```python
from build123d import *
from build123d.topology import SkipClean

# Parameters (mm, degrees)
BOSS_EXTRUDE1_DEPTH     = 2.5
BOSS_EXTRUDE1_2_DEPTH   = 2.5
BOSS_EXTRUDE2_DEPTH     = 6.35
BOSS_EXTRUDE3_DEPTH     = 6.35
SKETCH4_R               = 3.175
CUT_EXTRUDE1_DEPTH      = 25.4
SKETCH5_R               = 1.5875
CUT_EXTRUDE2_DEPTH      = 25.4
CUT_EXTRUDE3_DEPTH      = 25.4
CUT_EXTRUDE4_REACH      = 43
CUT_EXTRUDE4_END_RADIUS = 3.175
CUT_EXTRUDE5_REACH      = 39.36
SKETCH8_W               = 2.54
SKETCH8_H               = 9.525
SKETCH9_W               = 0.7112
SKETCH9_H               = 15.2
BOSS_EXTRUDE4_DEPTH     = 17
BOSS_EXTRUDE5_DEPTH     = 1.016
SKETCH11_W              = 1.176658287
SKETCH11_H              = 2.5
SKETCH11_W_2            = 2.636987944
SKETCH11_H_2            = 15.2
BOSS_EXTRUDE6_DEPTH     = 1.27
CUT_EXTRUDE6_DEPTH      = 38.864332241
BOSS_EXTRUDE7_START     = 2.54
BOSS_EXTRUDE7_DEPTH     = 2.54
BOSS_EXTRUDE8_DEPTH     = 2.54
BOSS_EXTRUDE9_DEPTH     = 0.508
BOSS_EXTRUDE10_DEPTH    = 0.508
CUT_EXTRUDE7_DEPTH      = 3.81
CUT_EXTRUDE8_DEPTH      = 3.81
BOSS_EXTRUDE11_DEPTH    = 3.81
BOSS_EXTRUDE12_START    = -10.16
SKETCH21_W              = 49.554714962
SKETCH21_H              = 15.2
SKETCH21_R              = 3.175
BOSS_EXTRUDE12_DEPTH    = 10.16


with BuildPart() as part:
    # Sketch1 → Boss-Extrude1 (new body)
    with BuildSketch(Plane.XY):
        Polygon((5.08, 0), (0, 0), (0, 19.141079028), (-1.033059908, 19.141079028), (-3.75575709, 23.125698967), (-8.376397661, 9.077684872), (-11.679025045, 6.820994294), (-21.26996, 20.857160675), (-22.86, 19.770683798), (-22.86, -3.81), (8.89, -3.81), (8.89, 24.384), (5.08, 24.384), align=None)
    extrude(amount=BOSS_EXTRUDE1_DEPTH)



with BuildPart() as body_2:
    # Sketch1 → Boss-Extrude1 2 (new body)
    with BuildSketch(Plane.XY):
        Polygon((-10.069369191, 23.749), (-4.328956497, 23.964566322), (-4.615556201, 24.384), (-16.108492032, 24.384), (-17.03780348, 23.749), align=None)
    extrude(amount=BOSS_EXTRUDE1_2_DEPTH)


with BuildPart() as part_1:
    add(part.part)

    add(body_2.part)  # Boss-Extrude2 merges body 2
    # Sketch2 → Boss-Extrude2 (add)
    with BuildSketch(Plane.XY.offset(2.5)):
        Polygon((-11.679025045, 6.820994294), (-21.26996, 20.857160675), (-22.86, 19.770683798), (-22.86, -3.81), (8.89, -3.81), (8.89, 24.384), (5.08, 24.384), (5.08, 0), (0, 0), (0, 19.141079028), (-1.033059908, 19.141079028), (-3.75575709, 23.125698967), (-8.376397661, 9.077684872), align=None)
        Polygon((-16.108492032, 24.384), (-18.00931945, 23.085161582), (-8.418384495, 9.048995201), (-8.376397661, 9.077684872), (-3.75575709, 23.125698967), (-1.033059908, 19.141079028), (0, 19.141079028), (0, 0), (5.08, 0), (5.08, 24.384), align=None)
    extrude(amount=BOSS_EXTRUDE2_DEPTH)

    # Sketch3 → Boss-Extrude3 (add)
    with BuildSketch(Plane(origin=(0, 0, 0), x_dir=(-1, 0, 0), z_dir=(0, 0, -1))):
        Polygon((-8.89, 24.384), (-8.89, -3.81), (22.86, -3.81), (22.86, 19.770683798), (21.26996, 20.857160675), (11.679025045, 6.820994294), (8.376397661, 9.077684872), (18.00931945, 23.085161582), (16.108492032, 24.384), align=None)
    extrude(amount=BOSS_EXTRUDE3_DEPTH)

    # Sketch4 → Cut-Extrude1 (cut)
    with BuildSketch(Plane(origin=(0, 24.384, 0), x_dir=(1, 0, 0), z_dir=(0, 1, 0))):
        with Locations(Location((2.54, -1.25, 0), (0, 0, 270))):
            Circle(SKETCH4_R)
    extrude(amount=-CUT_EXTRUDE1_DEPTH, mode=Mode.SUBTRACT)

    # Sketch5 → Cut-Extrude2 (cut)
    with BuildSketch(Plane(origin=(0, -1.016, 0), x_dir=(1, 0, 0), z_dir=(0, 1, 0))):
        with Locations(Location((2.54, -1.25, 0), (0, 0, 270))):
            Circle(SKETCH5_R)
    extrude(amount=-CUT_EXTRUDE2_DEPTH, mode=Mode.SUBTRACT)

    # Sketch6 → Cut-Extrude3 (cut)
    with BuildSketch(Plane.XY.offset(8.85)):
        Polygon((-22.86, 16.430904611), (-9.029357481, -3.81), (-22.86, -3.81), align=None)
    extrude(amount=-CUT_EXTRUDE3_DEPTH, mode=Mode.SUBTRACT)

    # Cut-Extrude4: up to this cylinder (the profile starts outside it)
    with SkipClean():  # the faces are left unmerged after this step: merging them gives an invalid solid
        cut_extrude4_end = Plane(origin=(2.54, 2.159, 1.25), z_dir=(0, 1, 0)) * Cylinder(CUT_EXTRUDE4_END_RADIUS, 96.045024, mode=Mode.PRIVATE)
        # Sketch7 → Cut-Extrude4 (cut, up to the surface)
        with BuildSketch(Plane(origin=(8.89, 0, 0), x_dir=(0, 0, -1), z_dir=(1, 0, 0)), mode=Mode.PRIVATE) as cut_extrude4_sk1:
            with BuildLine():
                ThreePointArc((1.925, 2.159), (-1.25, 5.334), (-4.425, 2.159))
                Line((-4.425, 2.159), (1.925, 2.159))
            make_face()
        cut_extrude4_tool1 = extrude(cut_extrude4_sk1.sketch, amount=-CUT_EXTRUDE4_REACH, mode=Mode.PRIVATE) - cut_extrude4_end
        add(cut_extrude4_tool1.solids().sort_by_distance((8.89, 3.506512, 1.25))[0], mode=Mode.SUBTRACT)
        # Sketch7 → Cut-Extrude4 (cut, up to the surface)
        with BuildSketch(Plane(origin=(8.89, 0, 0), x_dir=(0, 0, -1), z_dir=(1, 0, 0)), mode=Mode.PRIVATE) as cut_extrude4_sk2:
            with BuildLine():
                Line((1.925, 2.159), (-4.425, 2.159))
                ThreePointArc((-4.425, 2.159), (-3.49506403, -0.08606403), (-1.25, -1.016))
                ThreePointArc((-1.25, -1.016), (0.99506403, -0.08606403), (1.925, 2.159))
            make_face()
        cut_extrude4_tool2 = extrude(cut_extrude4_sk2.sketch, amount=-CUT_EXTRUDE4_REACH, mode=Mode.PRIVATE) - cut_extrude4_end
        add(cut_extrude4_tool2.solids().sort_by_distance((8.89, 0.811488, 1.25))[0], mode=Mode.SUBTRACT)
        # Sketch7 → Cut-Extrude4 (cut, up to the surface)
        with BuildSketch(Plane(origin=(8.89, 0, 0), x_dir=(0, 0, -1), z_dir=(1, 0, 0)), mode=Mode.PRIVATE) as cut_extrude4_sk3:
            with BuildLine():
                ThreePointArc((1.925, 2.159), (-1.25, 5.334), (-4.425, 2.159))
                Line((-4.425, 2.159), (1.925, 2.159))
            make_face()
        cut_extrude4_tool3 = extrude(cut_extrude4_sk3.sketch, amount=-CUT_EXTRUDE4_REACH, mode=Mode.PRIVATE) - cut_extrude4_end
        add(cut_extrude4_tool3.solids().sort_by_distance((8.89, 3.506512, 1.25))[0], mode=Mode.SUBTRACT)
        # Sketch7 → Cut-Extrude4 (cut, up to the surface)
        with BuildSketch(Plane(origin=(8.89, 0, 0), x_dir=(0, 0, -1), z_dir=(1, 0, 0)), mode=Mode.PRIVATE) as cut_extrude4_sk4:
            with BuildLine():
                Line((1.925, 2.159), (-4.425, 2.159))
                ThreePointArc((-4.425, 2.159), (-3.49506403, -0.08606403), (-1.25, -1.016))
                ThreePointArc((-1.25, -1.016), (0.99506403, -0.08606403), (1.925, 2.159))
            make_face()
        cut_extrude4_tool4 = extrude(cut_extrude4_sk4.sketch, amount=-CUT_EXTRUDE4_REACH, mode=Mode.PRIVATE) - cut_extrude4_end
        add(cut_extrude4_tool4.solids().sort_by_distance((8.89, 0.811488, 1.25))[0], mode=Mode.SUBTRACT)

    # Cut-Extrude5: up to this face of the body (flat: up to its plane)
    cut_extrude5_end = Plane(part_1.part.faces().sort_by_distance((4.72156403, -1.016, 3.43156403))[0])
    # Sketch8 → Cut-Extrude5 (cut, up to the picked face)
    with BuildSketch(Plane(origin=(0, 24.384, 0), x_dir=(1, 0, 0), z_dir=(0, 1, 0)), mode=Mode.PRIVATE) as cut_extrude5_sk1:
        with Locations((2.54, -1.25)):
            Rectangle(SKETCH8_W, SKETCH8_H)
    cut_extrude5_tool1 = split(extrude(cut_extrude5_sk1.sketch, amount=-CUT_EXTRUDE5_REACH, mode=Mode.PRIVATE), bisect_by=cut_extrude5_end, keep=Keep.BOTH, mode=Mode.PRIVATE)
    add(cut_extrude5_tool1.solids().sort_by(Axis((2.54, 24.384, 1.25), (0, -1, 0)))[0], mode=Mode.SUBTRACT)

    # Sketch9 → Boss-Extrude4 (add)
    with BuildSketch(Plane(origin=(-6.894633763, 10.090176515, 0), x_dir=(0.825656845959394, 0.5641726444275594, 0), z_dir=(-0.5641726444275594, 0.825656845959394, 0))):
        with Locations((-5.439048594, -1.25)):
            Rectangle(SKETCH9_W, SKETCH9_H)
        Polygon((-1.794648594, 6.35), (-2.302648594, 6.35), (-2.302648594, 1.6202), (-3.623501238, 1.6202), (-3.623501238, 0.7312), (-1.794648594, 0.7312), align=None)
        Polygon((-1.845501238, -8.85), (-1.845501238, -4.6028), (-3.572648594, -4.6028), (-3.572648594, -5.6188), (-2.683648594, -5.6188), (-2.683648594, -8.85), align=None)
    extrude(amount=BOSS_EXTRUDE4_DEPTH)

    # Sketch10 → Boss-Extrude5 (add)
    with BuildSketch(Plane(origin=(-6.894633763, 10.090176515, 0), x_dir=(0.8256568459593948, 0.5641726444275585, 0), z_dir=(-0.5641726444275585, 0.8256568459593948, 0))):
        Polygon((-5.083448594, -8.85), (-2.683648594, -8.85), (-2.683648594, -5.6188), (-3.572648594, -5.6188), (-3.572648594, -4.6028), (-1.845501238, -4.6028), (-1.845501238, -2.5), (-1.794648594, -2.5), (-1.794648594, 0), (-1.794648594, 0.7312), (-3.623501238, 0.7312), (-3.623501238, 1.6202), (-2.302648594, 1.6202), (-2.302648594, 6.35), (-5.083448594, 6.35), align=None)
    extrude(amount=BOSS_EXTRUDE5_DEPTH)

    # Sketch11 → Boss-Extrude6 (add)
    with BuildSketch(Plane(origin=(-16.485568719, 24.126342896, 0), x_dir=(0.8256568459593935, 0.5641726444275603, 0), z_dir=(-0.5641726444275603, 0.8256568459593935, 0))):
        with Locations((-1.257172095, -1.25)):
            Rectangle(SKETCH11_W, SKETCH11_H)
        Polygon((-3.623501238, 1.6202), (-3.623501238, 0.7312), (-1.845501238, 0.7312), (-1.845501238, 0), (-0.668842951, 0), (-0.668842951, -2.5), (-1.845501238, -2.5), (-1.845501238, -4.6028), (-3.572648594, -4.6028), (-3.572648594, -5.6188), (-2.683648594, -5.6188), (-2.683648594, -8.85), (0.456699038, -8.85), (0.456699038, 6.35), (-2.302648594, 6.35), (-2.302648594, 1.6202), align=None)
        with Locations((-6.401942566, -1.25)):
            Rectangle(SKETCH11_W_2, SKETCH11_H_2)
    extrude(amount=BOSS_EXTRUDE6_DEPTH)

    # Sketch12 → Cut-Extrude6 (cut, through all)
    with BuildSketch(Plane.XY.offset(8.85)):
        Polygon((-16.108492032, 24.384), (-18.359576008, 24.384), (-16.82499129, 25.432584194), align=None)
        Polygon((-22.86, 19.770683798), (-22.86, 21.308853083), (-23.576499258, 20.819267993), align=None)
    extrude(amount=-CUT_EXTRUDE6_DEPTH, mode=Mode.SUBTRACT)

    # Sketch13 → Boss-Extrude7 (add)
    with BuildSketch(Plane(origin=(0, 19.141079028, 0), x_dir=(1, 0, 0), z_dir=(0, 1, 0)).offset(BOSS_EXTRUDE7_START)):
        with BuildLine():
            Line((-0.378582704, 0), (-1.033059908, 0))
            Line((-1.033059908, 0), (-1.033059908, -2.5))
            Line((-1.033059908, -2.5), (-0.378582704, -2.5))
            ThreePointArc((-0.378582704, -2.5), (-0.635, -1.25), (-0.378582704, 0))
        make_face()
    extrude(amount=-BOSS_EXTRUDE7_DEPTH)

    # Sketch15 → Boss-Extrude8 (add)
    with BuildSketch(Plane.XY):
        Polygon((-4.156996675, 23.712906116), (-4.328956497, 23.964566322), (-4.808856613, 23.946544917), (-4.492543617, 23.483626353), align=None)
        Polygon((-3.75575709, 23.125698967), (-3.927716912, 23.377359173), (-4.263263855, 23.148079411), (-3.915700647, 22.639426706), align=None)
    extrude(amount=BOSS_EXTRUDE8_DEPTH)

    # Sketch16 → Boss-Extrude9 (add)
    with BuildSketch(Plane.XY):
        Polygon((-4.263263855, 23.148079411), (-4.492543617, 23.483626353), (-4.156996675, 23.712906116), (-3.927716912, 23.377359173), align=None)
    extrude(amount=BOSS_EXTRUDE9_DEPTH)

    # Sketch17 → Boss-Extrude10 (add)
    with BuildSketch(Plane(origin=(0, 0, 2.5), x_dir=(-1, 0, 0), z_dir=(0, 0, -1))):
        Polygon((4.263263855, 23.148079411), (4.492543617, 23.483626353), (4.156996675, 23.712906116), (3.927716912, 23.377359173), align=None)
    extrude(amount=BOSS_EXTRUDE10_DEPTH)

    # Sketch18 → Cut-Extrude7 (cut)
    with BuildSketch(Plane(origin=(0, 0, 2.5), x_dir=(-1, 0, 0), z_dir=(0, 0, -1))):
        Polygon((1.033059908, 24.384), (1.033059908, 21.681079028), (1.033059908, 19.141079028), (4.615556201, 24.384), align=None)
    extrude(amount=-CUT_EXTRUDE7_DEPTH, mode=Mode.SUBTRACT)

    # Sketch19 → Cut-Extrude8 (cut)
    with BuildSketch(Plane.XY):
        Polygon((-1.033059908, 19.141079028), (-1.033059908, 21.681079028), (-1.033059908, 24.384), (-4.615556201, 24.384), align=None)
    extrude(amount=-CUT_EXTRUDE8_DEPTH, mode=Mode.SUBTRACT)

    # Sketch20 → Boss-Extrude11 (add)
    with BuildSketch(Plane.XY):
        Polygon((-10.069369191, 23.749), (-4.492543617, 23.483626353), (-4.808856613, 23.946544917), align=None)
    extrude(amount=BOSS_EXTRUDE11_DEPTH)

    # Sketch21 → Boss-Extrude12 (add)
    with BuildSketch(Plane.XZ.offset(3.81).offset(BOSS_EXTRUDE12_START)):
        with Locations((15.748, 1.25)):
            Rectangle(SKETCH21_W, SKETCH21_H)
        with Locations(Location((2.54, 1.25, 0), (0, 0, 90))):
            Circle(SKETCH21_R, mode=Mode.SUBTRACT)
        with Locations(Location((28.956, 1.25, 0), (0, 0, 270))):
            Circle(SKETCH21_R, mode=Mode.SUBTRACT)
    extrude(amount=BOSS_EXTRUDE12_DEPTH)


solid = part_1.part
```
Here's how the part is built. I have some questions about the finished solid (model axes, mm). A direction names the side the tool comes from. Coordinates: 2 decimals unless noted, no trailing zeros. Loops run counter-clockwise (first coordinate to the right, second up) from the corner with the lowest first, then second, coordinate; pieces in that order, holes last. Notation, with made-up numbers: (25, 39.5) - (63, 39.5) arc R31 cw to (63, 76.5) - close; hole circle Ø1 at (-6, -26.5). An arc over 180 degrees is marked (long way). Return JSON: item names as keys, results as strings. Group by question number.
Item 1: We'd pull the mould along Y, two halves only. Please class faces 6 (the face through (16, -3.81, 1)), 7 (the face through (-22.14, 21.8, 1.14)), 8 (the face through (-13.42, 16.41, -0.36)), 9 (the face through (-22.86, 19, 1)): +Y half, -Y half, draft (parallel to the pull), parting line (faces both ways), or undercut.
Item 2: If we section it at C-C on y = 0.25: Write out the boundary of the cut face in (x, z) (3 decimals).
Item 3: Will these pins go through, and if not, where does the flat tip stop? P1, Ø5, axis at x = -15.5, y = 17.5, coming from the +Z side; P2, Ø1.2, axis at x = -15, z = 1, coming from the -Y side; P3, Ø12, axis at x = 32, y = 14, coming from the +Z side; P4, Ø3, axis at x = 2, z = 1.5, coming from the +Y side.
Item 4: I need wall thicknesses on line 1 (X direction, y = 21.75, z = -3.75); line 2 (X direction, y = 3.5, z = 1); line 3 (X direction, y = 19.5, z = 5.5). Which ranges of each line are inside material? Lowest first, please. Write a range as from..to.
Item 5: If we section it at B-B on x = 30: Write out the boundary of the cut face in (y, z).
Item 6: On a 3-axis mill with a long thin cutter (end or side, diameter ignored), from which of +Z, -Z, +X, -X, +Y, -Y can I reach the whole of each face in a straight line? I mean faces 1 (the face through (-16.46, 15.08, 1.36)), 2 (the face through (1.27, 15, -3)), 3 (the face through (-11, 20, 0)), 4 (the face through (8.89, 15, 1)), 5 (the face through (-16.04, 6.45, 1.36)). Say none if no direction works.
Item 7: If we section it at A-A on y = 18.25: State how many separate pieces and enclosed holes the cut face has, and give its area (3 significant figures).
Calculated:
{
 "1": {"face 6": "-Y half", "face 7": "+Y half", "face 8": "undercut", "face 9": "draft"},
 "2": {"outline": "(-11.804, -6.35) - (40.525, -6.35) - (40.525, 8.85) - (-11.804, 8.85) - close; hole circle Ø6.35 at (2.54, 1.25); hole circle Ø6.35 at (28.956, 1.25)"},
 "3": {"P1": "stops at z = 8.85", "P2": "stops at y = 4.05", "P3": "passes through", "P4": "stops at y = -1.02"},
 "4": {"line 1": "x = -22.21..-21.02, -17.65..-2.82, -1.03..8.89", "line 2": "x = -14.02..-0.63, 5.71..25.79, 32.12..40.53", "line 3": "x = -22.86..-19.48, -17.65..-1.28, -1.03..1.27, 3.81..8.89"},
 "5": {"outline": "(-3.81, -6.35) - (6.35, -6.35) - (6.35, -1.75) - (-3.81, -1.75) - close; (-3.81, 4.25) - (6.35, 4.25) - (6.35, 8.85) - (-3.81, 8.85) - close"},
 "6": {"face 1": "+Z, -Z", "face 2": "+Y", "face 3": "none", "face 4": "+Z, -Z, +X, +Y", "face 5": "+Z, -Z, -X, -Y"},
 "7": {"separate pieces": "2", "enclosed holes": "1", "area": "369 mm^2"}
}
